Verification items for the finished model (mm, model axes). A direction names the side the tool comes from. Round coordinates to 2 decimals unless told otherwise and drop trailing zeros. Order: outer loops, then holes, each group sorted by start corner. A loop starts at its lowest first (then second) coordinate and runs counter-clockwise, first axis right, second up. Notation, with made-up numbers: (22.5, 77.25) -> (34.5, 77.25) arc R21 cw to (34.5, 108.25) -> close; hole circle Ø3 at (-7.75, -28). An arc over 180 degrees is marked (long way). Write item = value, one per line. Start each with the question number.
from build123d import *

# Parameters (mm, degrees)
F1_DEPTH = 10
F3_D     = 10


with BuildPart() as f1:
    # F0 (on Top) → F1 (new body)
    with BuildSketch(Plane.XY):
        with BuildLine():
            Line((10, -100), (10, 0))
            ThreePointArc((10, 0), (0, 10), (-10, 0))
            Line((-10, 0), (-10, -100))
            ThreePointArc((-10, -100), (0, -110), (10, -100))
        make_face()
        with BuildLine():
            ThreePointArc((-5, -30), (0, -25), (5, -30))
            Line((5, -30), (5, -70))
            ThreePointArc((5, -70), (0, -75), (-5, -70))
            Line((-5, -70), (-5, -30))
        make_face(mode=Mode.SUBTRACT)
    extrude(amount=F1_DEPTH)

    # F3 (through all)
    with Locations(Plane.XY.offset(10)):
        with Locations((0, 0), (0, -100)):
            Hole(F3_D / 2)


solid = f1.part
(1) Depth check by flat-ended pin: pin 1 (1 mm diameter, centred on x = -3.5, z = 2, fed in from -Y). Enter the tip coordinate at first touch or a pass-through.
(2) Draft check along Y on faces 1 (the cylindrical face through (0, -110, 5)), 2 (the cylindrical face through (0, 10, 5)), 3 (the flat face through (-5, -50, 5)). Enter one of: +Y half, -Y half, draft (parallel to the pull), parting line (faces both ways), or undercut.
(3) Set-up check for faces 4 (the flat face through (10, -51, 5)), 5 (the cylindrical face through (0, -75, 5)): record each of +Z, -Z, +X, -X, +Y, -Y from which the full face is reachable in a straight line by a thin tool's end or side.
(4) Cross-section at B-B (y = -48). Enter the section's corners in (x, z), and give its area (3 significant figures).
(5) Cross-section at A-A (x = 0). Enter the section's corners in (y, z), and give its area (3 significant figures).
(6) Scan lines: line 1 along Y through (x, z) = (0, 6.5); line 2 along X through (y, z) = (-39, 5.5); line 3 along Y through (x, z) = (2, 4.5). Record each from-to range of solid material in increasing order. Write a range as from..to.
(7) Cross-section at D-D (y = -27). Enter the section's corners in (x, z), and give its area (3 significant figures).
(8) Cross-section at C-C (z = 8.25). Enter the section's corners in (x, y).
Outcome:
q1.pin_1 = -109.54
q2.face_1 = -Y half
q2.face_2 = +Y half
q2.face_3 = undercut
q3.face_4 = +Z, -Z, +X, +Y, -Y
q3.face_5 = +Z, -Z
q4.outline = (-10, 0) -> (-5, 0) -> (-5, 10) -> (-10, 10) -> close; (5, 0) -> (10, 0) -> (10, 10) -> (5, 10) -> close
q4.area = 100 mm^2
q5.outline = (-110, 0) -> (-105, 0) -> (-105, 10) -> (-110, 10) -> close; (-95, 0) -> (-75, 0) -> (-75, 10) -> (-95, 10) -> close; (-25, 0) -> (-5, 0) -> (-5, 10) -> (-25, 10) -> close; (5, 0) -> (10, 0) -> (10, 10) -> (5, 10) -> close
q5.area = 500 mm^2
q6.line_1 = -110..-105, -95..-75, -25..-5, 5..10
q6.line_2 = -10..-5, 5..10
q6.line_3 = -109.8..-104.58, -95.42..-74.58, -25.42..-4.58, 4.58..9.8
q7.outline = (-10, 0) -> (-4, 0) -> (-4, 10) -> (-10, 10) -> close; (4, 0) -> (10, 0) -> (10, 10) -> (4, 10) -> close
q7.area = 120 mm^2
q8.outline = (-10, -100) arc R10 ccw to (10, -100) -> (10, 0) arc R10 ccw to (-10, 0) -> close; hole circle Ø10 at (0, -100); hole (-5, -70) arc R5 ccw to (5, -70) -> (5, -30) arc R5 ccw to (-5, -30) -> close; hole circle Ø10 at (0, 0)
